```python
from build123d import *

# Parameters (mm, degrees)
F0_W     = 609.6
F0_H     = 228.6
F1_DEPTH = 863.6
F2_W     = 95.25
F2_H     = 622.3
F3_DEPTH = 25.4
F4_R     = 5.08
F5_W     = 228.6
F5_H     = 101.6
F6_DEPTH = 76.2
F7_W     = 228.6
F7_H     = 778.857014
F7_W_2   = 209.296
F7_H_2   = 759.553014
F8_DEPTH = 15.875


with BuildPart() as f1:
    # F0 (on Top) → F1 (new body)
    with BuildSketch(Plane.XY):
        with Locations((-304.8, 114.3)):
            Rectangle(F0_W, F0_H)
    extrude(amount=F1_DEPTH)

    # F2 (on face) → F3 (cut)
    with BuildSketch(Plane.YZ):
        with Locations((111.125, 482.6)):
            Rectangle(F2_W, F2_H)
    extrude(amount=-F3_DEPTH, mode=Mode.SUBTRACT)

    # F4
    f4_edges = [f1.edges().sort_by_distance(p)[0] for p in [
        (-25.4, 158.75, 482.6),
        (-25.4, 111.125, 793.75),
        (-25.4, 63.5, 482.6),
        (-25.4, 111.125, 171.45),
    ]]
    fillet(f4_edges, radius=F4_R)

    # F5 (on face) → F6 (cut)
    with BuildSketch(Plane.YZ):
        with Locations((114.3, 50.8)):
            Rectangle(F5_W, F5_H)
    extrude(amount=-F6_DEPTH, mode=Mode.SUBTRACT)

    # F7 (on face) → F8 (cut)
    with BuildSketch(Plane.YZ):
        with Locations((114.3, 474.171493)):
            Rectangle(F7_W, F7_H)
        with Locations((114.3, 474.171493)):
            Rectangle(F7_W_2, F7_H_2, mode=Mode.SUBTRACT)
    extrude(amount=-F8_DEPTH, mode=Mode.SUBTRACT)


solid = f1.part
```
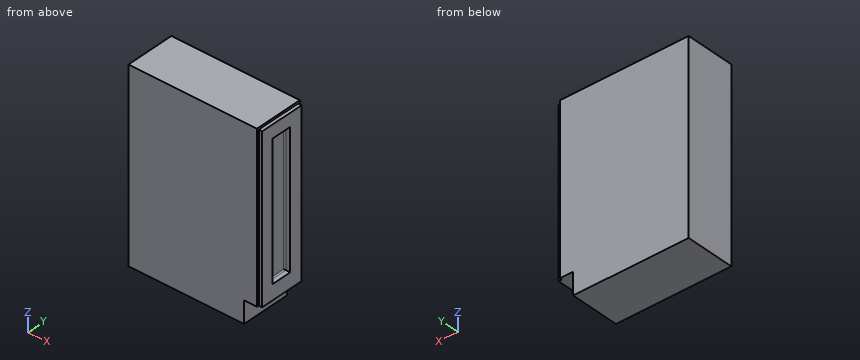
Can you work these out from the model? Positions are in its coordinate system, mm. Give positions to 0.01 mm unless a question says otherwise; leave off trailing zeros. Loops run counter-clockwise (first coordinate to the right, second up) from the corner with the lowest first, then second, coordinate; pieces in that order, holes last. Notation, with made-up numbers: M 54,-31.5 L 61,-31.5 A15 cw 61,-3.5 Z; hole C -28,-37.75 d6. An arc over 180 degrees is marked long. One line per item, written item: value.
(1) I need wall thicknesses on line 1 (X direction, y = 126.5, z = 330.5); line 2 (X direction, y = 83.5, z = 44); line 3 (Z direction, x = -74, y = 135.5). Which ranges of each line are inside material? Lowest first, please.
Returned:
line 1: -609.6 to -25.4
line 2: -609.6 to -76.2
line 3: 101.6 to 863.6
(2) Will these pins go through, and if not, where does the flat tip stop? pin 1 (22.5 mm diameter, centred on x = -7, y = 107.5, fed in from -Z); pin 2 (10 mm diameter, centred on x = -8, z = 613.5, fed in from +Y); pin 3 (5 mm diameter, centred on y = 99.5, z = 434, fed in from +X).
Returned:
pin 1: z = 101.6
pin 2: y = 218.95
pin 3: x = -25.4
(3) Suppose I cut it at B-B on y = 138. List the corners of the cut face in (x, z) for me (3 decimals), plus the area to 3 significant figures.
Returned:
outline: M -609.6,0 L -76.2,0 L -76.2,101.6 L 0,101.6 L 0,171.45 L -20.32,171.45 A5.08 cw -25.4,176.53 L -25.4,788.67 A5.08 cw -20.32,793.75 L 0,793.75 L 0,853.948 L -15.875,853.948 L -15.875,863.6 L -609.6,863.6 Z
area: 503,000 mm^2
(4) Suppose I cut it at C-C on z = 59.5. List the corners of the cut face in (x, y) for me.
Returned:
outline: M -609.6,0 L -76.2,0 L -76.2,228.6 L -609.6,228.6 Z
(5) Suppose I cut it at A-A on z = 553.5. List the corners of the cut face in (x, y) for me (3 decimals), plus the area to 3 significant figures.
Returned:
outline: M -609.6,0 L -15.875,0 L -15.875,9.652 L 0,9.652 L 0,63.5 L -20.32,63.5 A5.08 cw -25.4,68.58 L -25.4,153.67 A5.08 cw -20.32,158.75 L 0,158.75 L 0,218.948 L -15.875,218.948 L -15.875,228.6 L -609.6,228.6 Z
area: 137,000 mm^2
